```python
from build123d import *

# Parameters (mm, degrees)
SKETCH_1_R      = 25
EXTRUDE_1_DEPTH = 230
SKETCH_2_W      = 230
SKETCH_2_H      = 70
EXTRUDE_2_DEPTH = 18
SKETCH_3_W      = 223
SKETCH_3_H      = 120
EXTRUDE_3_DEPTH = 30
EXTRUDE_4_DEPTH = 3
SKETCH_5_R      = 25
EXTRUDE_5_DEPTH = 8


with BuildPart() as part:
    # 草图1 → 凸台-拉伸1 (new body)
    with BuildSketch(Plane.XY):
        with BuildLine():
            Line((0, 50), (150, 50))
            Line((150, 50), (150, -50))
            Line((150, -50), (0, -50))
            ThreePointArc((0, -50), (-50, 0), (0, 50))
        make_face()
        Circle(SKETCH_1_R, mode=Mode.SUBTRACT)
    extrude(amount=EXTRUDE_1_DEPTH)

    # 草图2 → 凸台-拉伸2 (add)
    with BuildSketch(Plane(origin=(150, 0, 0), x_dir=(0, 0, -1), z_dir=(1, 0, 0))):
        with Locations((-115, 0)):
            Rectangle(SKETCH_2_W, SKETCH_2_H)
    extrude(amount=EXTRUDE_2_DEPTH)

    # 草图3 → 凸台-拉伸3 (add)
    with BuildSketch(Plane(origin=(0, 0, 0), x_dir=(-1, 0, 0), z_dir=(0, 0, -1))):
        with Locations((-56.5, 0)):
            Rectangle(SKETCH_3_W, SKETCH_3_H)
    extrude(amount=-EXTRUDE_3_DEPTH)

    # 草图4 → 凸台-拉伸4 (add)
    with BuildSketch(Plane.XY.offset(230)):
        with BuildLine():
            Line((168, 25), (141, 25))
            ThreePointArc((141, 25), (116, 0), (141, -25))
            Line((141, -25), (168, -25))
            Line((168, -25), (168, 25))
        make_face()
    extrude(amount=EXTRUDE_4_DEPTH)

    # 草图5 → 凸台-拉伸5 (add)
    with BuildSketch(Plane.XY.offset(230)):
        with BuildLine():
            Line((-55.646359671, 10), (-55.646359671, -10))
            Line((-55.646359671, -10), (-33.541019662, -10))
            ThreePointArc((-33.541019662, -10), (-17.5, -30.310889132), (8.110255793, -34.047375097))
            Line((8.110255793, -34.047375097), (19.162925798, -53.191161103))
            Line((19.162925798, -53.191161103), (36.483433873, -43.191161103))
            Line((36.483433873, -43.191161103), (25.430763869, -24.047375097))
            ThreePointArc((25.430763869, -24.047375097), (35, 0), (25.430763869, 24.047375097))
            Line((25.430763869, 24.047375097), (36.483433873, 43.191161103))
            Line((36.483433873, 43.191161103), (19.162925798, 53.191161103))
            Line((19.162925798, 53.191161103), (8.110255793, 34.047375097))
            ThreePointArc((8.110255793, 34.047375097), (-17.5, 30.310889132), (-33.541019662, 10))
            Line((-33.541019662, 10), (-55.646359671, 10))
        make_face()
        Circle(SKETCH_5_R, mode=Mode.SUBTRACT)
    extrude(amount=EXTRUDE_5_DEPTH)


solid = part.part
```
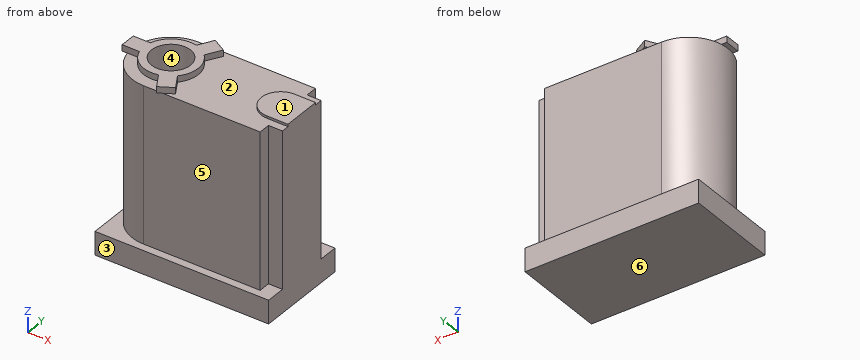
Model file for the job. Use its own axes, mm. Face numbers are marked on the shaded views. A direction names the side the tool comes from. Give positions to 0.01 mm unless a question says otherwise; leave off trailing zeros. Order: outer loops, then holes, each group sorted by start corner. A loop starts at its lowest first (then second) coordinate and runs counter-clockwise, first axis right, second up.
1) Saw through at A-A, the plane z = 90.5. Write the cut outline in (x, y), then the cut area to 3 significant figures.
2) Saw through at D-D, the plane x = 41.5. Write the cut outline in (y, z).
3) Mould opens along Y. For the marked faces 4, 5 and 6 say: +Y half, -Y half, draft (parallel to the pull), parting line (faces both ways), or undercut.
4) Wall check: probe 1 along Y at (x, z) = (0, 174); probe 2 along X at (y, z) = (0, 146); probe 3 along Y at (x, z) = (66, 112.5). Give the ranges that are in metal, low to high.
5) 3-axis set-ups, long thin cutter, end or side, ignore diameter. For the marked faces 1, 2 and 3: which of +Z, -Z, +X, -X, +Y, -Y reach the whole face in a straight line?
6) Pin check, flat tips, straight feed: pin 1 (5 mm diameter, centred on x = -23, z = 62.5, fed in from +Y); pin 2 (12 mm diameter, centred on x = -18.5, z = 214, fed in from -Y); pin 3 (10 mm diameter, centred on y = 42.5, z = 80, fed in from +X). Stop position of each tip, or through.
7) Saw through at B-B, the plane y = 0. Write the cut outline in (x, z), then the cut area to 3 significant figures.
8) Saw through at C-C, the plane x = 130. Write the cut outline in (y, z).
Computed:
1. outline: (0, -50) - (150, -50) - (150, -35) - (168, -35) - (168, 35) - (150, 35) - (150, 50) - (0, 50) arc R50 ccw to start; hole circle Ø50 at (0, 0)
1. area: 18,200 mm2
2. outline: (-60, 0) - (60, 0) - (60, 30) - (50, 30) - (50, 230) - (-50, 230) - (-50, 30) - (-60, 30) - close
3. face 4: undercut
3. face 5: -Y half
3. face 6: draft
4. probe 1: y = -50 to -25, 25 to 50
4. probe 2: x = -50 to -25, 25 to 168
4. probe 3: y = -50 to 50
5. face 1: +Z, +X, +Y, -Y
5. face 2: +Z
5. face 3: +Z, -Z, +X, -X, -Y
6. pin 1: stops at y = 45.6
6. pin 2: stops at y = -48.41
6. pin 3: stops at x = 150
7. outline: (-55.65, 230) - (-50, 230) - (-50, 30) - (-55, 30) - (-55, 0) - (168, 0) - (168, 233) - (116, 233) - (116, 230) - (35, 230) - (35, 238) - (25, 238) - (25, 30) - (-25, 30) - (-25, 238) - (-55.65, 238) - close
7. area: 40,800 mm2
8. outline: (-60, 0) - (60, 0) - (60, 30) - (50, 30) - (50, 230) - (22.45, 230) - (22.45, 233) - (-22.45, 233) - (-22.45, 230) - (-50, 230) - (-50, 30) - (-60, 30) - close
